from build123d import *

# Parameters (mm, degrees)
F0_R             = 7.6394373987
F0_R_2           = 4.25
F1_DEPTH         = 11
F3_DEPTH         = 11.001
F3_COPIES_COUNT  = 8
F3_COPIES_ANGLE  = 157.5
F3_COPIES1_COUNT = 9
F3_COPIES1_ANGLE = 180
F4_R             = 8
F4_R_2           = 4.25
F5_DEPTH         = 1
F6_R             = 4.25
F7_DEPTH         = 8
F8_R             = 1.9
F9_DEPTH         = 10


# Not quite as in the source:
# - ends of sketch curves that miss each other by under 0.0002 mm in the source are joined
# - a pattern or mirror of a feature is missing from the dataset's text; its kind, count and spacing are read off the source's solid
# - a feature names something its author has since deleted; it is built from what else it names


with BuildPart() as f1:
    # F0 (on Top) → F1 (new body)
    with BuildSketch(Plane.XY):
        Circle(F0_R)
        Circle(F0_R_2, mode=Mode.SUBTRACT)
    extrude(amount=F1_DEPTH)

    # F2 (on Top) → F3 (cut, through all)
    with BuildSketch(Plane.XY):
        with BuildLine():
            ThreePointArc((0.9017719181, -7.0023415032), (0.5987456618, -6.4391610804), (0, -6.2144373987))
            ThreePointArc((0, -6.2144373987), (-0.5987456618, -6.4391610804), (-0.9017719181, -7.0023415032))
            ThreePointArc((-0.9017719181, -7.0023415032), (-0.9975198669, -7.184187159), (-1.1896796808, -7.25699))
            Line((-1.1896796808, -7.25699), (-2.3868598428, -7.25699))
            ThreePointArc((-2.3868598428, -7.25699), (0, -7.6394373987), (2.3868598428, -7.25699))
            Line((2.3868598428, -7.25699), (1.1896796808, -7.25699))
            ThreePointArc((1.1896796808, -7.25699), (0.9975198669, -7.184187159), (0.9017719181, -7.0023415032))
        make_face()
    f3 = extrude(amount=F3_DEPTH, mode=Mode.SUBTRACT)

    # F3_copies: F3 ×8 about axis
    f3_copies_axis = Axis((0, 0, 0), (0, 0, -1))
    for i in range(1, F3_COPIES_COUNT):
        add(f3.rotate(f3_copies_axis, i * F3_COPIES_ANGLE / (F3_COPIES_COUNT - 1)), mode=Mode.SUBTRACT)

    # F3_copies1: F3 ×9 about axis
    f3_copies1_axis = Axis((0, 0, 0), (0, 0, 1))
    for i in range(1, F3_COPIES1_COUNT):
        add(f3.rotate(f3_copies1_axis, i * F3_COPIES1_ANGLE / (F3_COPIES1_COUNT - 1)), mode=Mode.SUBTRACT)

    # F4 (on face) → F5 (join)
    with BuildSketch(Plane(origin=(0, 0, 0), x_dir=(1, 0, 0), z_dir=(0, 0, -1))):
        Circle(F4_R)
        Circle(F4_R_2, mode=Mode.SUBTRACT)
    extrude(amount=F5_DEPTH)

    # F6 (on face) → F7 (join)
    with BuildSketch(Plane.XY.offset(11)):
        with BuildLine():
            Line((-5.5, 4.2538924505), (-5.5, 0))
            ThreePointArc((-5.5, 0), (0, -5.5), (5.5, 0))
            Line((5.5, 0), (5.5, 4.2538924505))
            ThreePointArc((5.5, 4.2538924505), (4.3574531497, 4.4333271044), (4.3137541227, 5.5890521994))
            ThreePointArc((4.3137541227, 5.5890521994), (4.3746351807, 5.7853277116), (4.2902362702, 5.9726974098))
            Line((4.2902362702, 5.9726974098), (4.1107546227, 6.1521790573))
            Line((4.1107546227, 6.1521790573), (3.8762505492, 6.249313825))
            ThreePointArc((3.8762505492, 6.249313825), (3.8754150111, 6.2496582146), (3.8745784043, 6.25))
            Line((3.8745784043, 6.25), (3.6559571933, 6.25))
            ThreePointArc((3.6559571933, 6.25), (3.5737630913, 6.1992003777), (3.5128086992, 6.1242268216))
            ThreePointArc((3.5128086992, 6.1242268216), (2.65655008, 5.6748069492), (1.8791762967, 6.25))
            Line((1.8791762967, 6.25), (0.2519111663, 6.25))
            ThreePointArc((0.2519111663, 6.25), (0, 6.2144373987), (-0.2519111663, 6.25))
            Line((-0.2519111663, 6.25), (-1.8791762967, 6.25))
            ThreePointArc((-1.8791762967, 6.25), (-2.65655008, 5.6748069492), (-3.5128086992, 6.1242268216))
            ThreePointArc((-3.5128086992, 6.1242268216), (-3.5737630913, 6.1992003777), (-3.6559571933, 6.25))
            Line((-3.6559571933, 6.25), (-3.8745784043, 6.25))
            ThreePointArc((-3.8745784043, 6.25), (-3.8754150111, 6.2496582146), (-3.8762505492, 6.249313825))
            Line((-3.8762505492, 6.249313825), (-4.1107546227, 6.1521790573))
            Line((-4.1107546227, 6.1521790573), (-4.2902362702, 5.9726974098))
            ThreePointArc((-4.2902362702, 5.9726974098), (-4.3746351807, 5.7853277116), (-4.3137541227, 5.5890521994))
            ThreePointArc((-4.3137541227, 5.5890521994), (-4.3574531497, 4.4333271044), (-5.5, 4.2538924505))
        make_face()
        Circle(F6_R, mode=Mode.SUBTRACT)
        with BuildLine():
            Line((-5.5, 11.55), (-5.5, 4.2538924505))
            ThreePointArc((-5.5, 4.2538924505), (-4.3574531497, 4.4333271044), (-4.3137541227, 5.5890521994))
            ThreePointArc((-4.3137541227, 5.5890521994), (-4.3746351807, 5.7853277116), (-4.2902362702, 5.9726974098))
            Line((-4.2902362702, 5.9726974098), (-4.1107546227, 6.1521790573))
            Line((-4.1107546227, 6.1521790573), (-3.8762505492, 6.249313825))
            ThreePointArc((-3.8762505492, 6.249313825), (-3.8754150111, 6.2496582146), (-3.8745784043, 6.25))
            Line((-3.8745784043, 6.25), (-4, 6.25))
            Line((-4, 6.25), (-4, 10.05))
            Line((-4, 10.05), (4, 10.05))
            Line((4, 10.05), (4, 6.25))
            Line((4, 6.25), (3.8745784043, 6.25))
            ThreePointArc((3.8745784043, 6.25), (3.8754150111, 6.2496582146), (3.8762505492, 6.249313825))
            Line((3.8762505492, 6.249313825), (4.1107546227, 6.1521790573))
            Line((4.1107546227, 6.1521790573), (4.2902362702, 5.9726974098))
            ThreePointArc((4.2902362702, 5.9726974098), (4.3746351807, 5.7853277116), (4.3137541227, 5.5890521994))
            ThreePointArc((4.3137541227, 5.5890521994), (4.3574531497, 4.4333271044), (5.5, 4.2538924505))
            Line((5.5, 4.2538924505), (5.5, 11.55))
            Line((5.5, 11.55), (-5.5, 11.55))
        make_face()
        with BuildLine():
            Line((-1.8791762967, 6.25), (-3.6559571933, 6.25))
            ThreePointArc((-3.6559571933, 6.25), (-3.5737630913, 6.1992003777), (-3.5128086992, 6.1242268216))
            ThreePointArc((-3.5128086992, 6.1242268216), (-2.65655008, 5.6748069492), (-1.8791762967, 6.25))
        make_face()
        with BuildLine():
            ThreePointArc((3.5128086992, 6.1242268216), (3.5737630913, 6.1992003777), (3.6559571933, 6.25))
            Line((3.6559571933, 6.25), (1.8791762967, 6.25))
            ThreePointArc((1.8791762967, 6.25), (2.65655008, 5.6748069492), (3.5128086992, 6.1242268216))
        make_face()
    extrude(amount=F7_DEPTH)

    # F8 (on face) → F9 (cut)
    with BuildSketch(Plane(origin=(0, 11.55, 0), x_dir=(-1, 0, 0), z_dir=(0, 1, 0))):
        with Locations((0, 15.5)):
            Circle(F8_R)
    extrude(amount=-F9_DEPTH, mode=Mode.SUBTRACT)


solid = f1.part
Geometry: final body of the model. Coordinates: model frame, mm. A direction names the side the tool comes from. Give positions to 0.01 mm unless a question says otherwise; leave off trailing zeros. Loops run counter-clockwise (first coordinate to the right, second up) from the corner with the lowest first, then second, coordinate; pieces in that order, holes last. Notation, with made-up numbers: M -15,45 L 39,45 A21 ccw 39,52 Z; hole C 61.5,-18 d11. An arc over 180 degrees is marked long. Put each result on its own line as item: value. Start each with the question number.
1) Access query for faces 4 (the flat face through (-5.5, 6, 15)), 5 (the flat face through (-3, 6.25, 15)), 6 (the cylindrical face through (-1.755, 5.043, 14.772)), 7 (the flat face through (0, -6, 11)), 8 (the flat face through (5.5, 6, 15)). Directions: +Z, -Z, +X, -X, +Y, -Y. A direction counts if a zero-diameter tool reaches every point of the face in a straight line with its end or side. Return the directions, or none.
2) Pull-direction query (Z, two-part tool) for faces 1 (the flat face through (0, 10.05, 13)), 2 (the flat face through (0, 5, 19)), 3 (the cylindrical face through (0.247, 10.811, 17.384)); classes: pulls with the +Z half, pulls with the -Z half, needs draft (parallel to the pull), parting line crosses it, or undercut.
3) Cut plane C-C (y = -2.75). Output: boundary loops of the cut face in (x, z), then the cut area to 3 significant figures.
4) Contact query for flat-ended pins moving along their axis: pin 1 (10 mm diameter, centred on y = 3, z = 13.5, fed in from -X); pin 2 (4 mm diameter, centred on x = 1.5, z = 15.5, fed in from -Y); pin 3 (6 mm diameter, centred on y = 4.5, z = 10, fed in from -X). Output: stop coordinate, or through.
5) Cut plane A-A (z = 12). Output: boundary loops of the cut face in (x, y).
6) Ray query, line 1 along Z through (x, y) = (0, 11.1); line 2 along X through (y, z) = (0, 8.5); line 3 along X through (y, z) = (4.8, 15.5). Return the intervals inside material, ascending.
7) Cut plane B-B (z = 15.5). Output: boundary loops of the cut face in (x, y), then the cut area to 3 significant figures.
Verdict:
1. face 4: +Z, -X, +Y, -Y
1. face 5: +Z
1. face 6: +Y
1. face 7: +Z, -Y
1. face 8: +Z, +X, +Y, -Y
2. face 1: needs draft
2. face 2: pulls with the +Z half
2. face 3: undercut
3. outline: M -7.51,-1 L -3.24,-1 L -3.24,19 L -4.76,19 L -4.76,11 L -5.67,11 L -5.67,0 L -7.51,0 Z; M 3.24,-1 L 7.51,-1 L 7.51,0 L 5.67,0 L 5.67,11 L 4.76,11 L 4.76,19 L 3.24,19 Z
3. area: 86.4 mm2
4. pin 1: x = -7.26
4. pin 2: y = -5.5
4. pin 3: x = -7.23
5. outline: M -5.5,0 A5.5 ccw 5.5,0 L 5.5,11.55 L -5.5,11.55 Z; hole C 0,0 d8.5; hole M -4,6.25 L -0.25,6.25 A0.91 ccw 0.25,6.25 L 4,6.25 L 4,10.05 L -4,10.05 Z
6. line 1: 11 to 13.6, 17.4 to 19
6. line 2: -6.21 to -4.25, 4.25 to 6.21
6. line 3: -5.5 to -1.9, 1.9 to 5.5
7. outline: M -5.5,0 A5.5 ccw 5.5,0 L 5.5,11.55 L 1.9,11.55 L 1.9,10.05 L 4,10.05 L 4,6.25 L 1.9,6.25 L 1.9,3.8 A4.25 cw long -1.9,3.8 L -1.9,6.25 L -4,6.25 L -4,10.05 L -1.9,10.05 L -1.9,11.55 L -5.5,11.55 Z
7. area: 73.6 mm2
